The model under review builds one solid part; all positions refer to its coordinate system, in mm. A direction names the side the tool comes from. Coordinates: 2 decimals unless noted, no trailing zeros. Order: outer loops, then holes, each group sorted by start corner. A loop starts at its lowest first (then second) coordinate and runs counter-clockwise, first axis right, second up. Notation, with made-up numbers: M -12,-22.75 L 22,-22.75 A26 ccw 22,16.25 Z; hole C 69.25,74.5 d1. An arc over 180 degrees is marked long. Answer as CSV lines item,"result". Start each with the question number.
Q1. Consider section B-B on y = 7. Write out the cut boundary in (x, z), and give its area (3 significant figures).
Q2. The part is to be moulded in two halves that separate along Y. For faces 1 (the face through (23.846, 7.509, -29.58)), 2 (the face through (17, -2, -4)), 3 (the face through (0, 0, -100)), say which applies: +Y half, -Y half, draft (parallel to the pull), parting line (faces both ways), or undercut.
Q3. Consider section D-D on x = 0. Write out the cut boundary in (y, z).
Q4. Wall thickness on L1, parallel to Z at x = 23.5, y = 6.5; L2, parallel to X at y = -5.5, z = -8; L3, parallel to X at y = 15, z = -71: over which ranges is each line inside the solid? List them lowest first. Write a range as [from, to].
Q5. Consider section C-C on z = -31.5. Write out the cut boundary in (x, y), and give its area (3 significant figures).
Q6. For P1, Ø3, axis at y = -3, z = -1.5, coming from the +X side; P2, Ø2, axis at x = 20, z = -2, coming from the -Y side; P3, Ø1.2, axis at x = 17.5, y = -2.5, coming from the +Z side; P4, Ø1, axis at x = 7.5, y = 3, coming from the +Z side, all flat-tipped, find the tip position at first contact; note any pin that passes through.
Q7. Machinability: for faces 4 (the face through (11, -16, -60)), 5 (the face through (0, 0, 0)), 6 (the face through (17, 0, -2)), which of the approach directions +Z, -Z, +X, -X, +Y, -Y give a long, thin tool a straight path to every point of the face, cutting with its end or side? Answer none if there is none.
Q8. Consider section A-A on x = 13. Write out the cut boundary in (y, z).
from build123d import *

# Parameters (mm, degrees)
SKETCH_1_R          = 25
EXTRUDE_1_DEPTH     = 60
SKETCH_2_R          = 18
EXTRUDE_2_DEPTH     = 100
SKETCH_3_W          = 25
SKETCH_3_H          = 8
CUT_EXTRUDE_1_DEPTH = 4


with BuildPart() as part:
    # 草图1 → 凸台-拉伸1 (new body)
    with BuildSketch(Plane.XY):
        Circle(SKETCH_1_R)
    extrude(amount=-EXTRUDE_1_DEPTH)

    # 草图2 → 凸台-拉伸2 (add)
    with BuildSketch(Plane.XY):
        Circle(SKETCH_2_R)
    extrude(amount=-EXTRUDE_2_DEPTH)

    # 草图3 → 切除-拉伸1 (cut)
    with BuildSketch(Plane(origin=(0, 0, 0), x_dir=(1, 0, 0), z_dir=(0, 1, 0))):
        with Locations((22.5, 0)):
            Rectangle(SKETCH_3_W, SKETCH_3_H)
    extrude(amount=-CUT_EXTRUDE_1_DEPTH, mode=Mode.SUBTRACT)


solid = part.part
Evaluation:
1,outline,"M -24,-60 L -16.58,-60 L -16.58,-100 L 16.58,-100 L 16.58,-60 L 24,-60 L 24,0 L -24,0 Z"
1,area,"4,210 mm²"
2,face 1,"parting line"
2,face 2,"undercut"
2,face 3,"draft"
3,outline,"M -25,-60 L -18,-60 L -18,-100 L 18,-100 L 18,-60 L 25,-60 L 25,0 L -25,0 Z"
4,L1,"z = [-60, 0]"
4,L2,"x = [-24.39, 24.39]"
4,L3,"x = [-9.95, 9.95]"
5,outline,"C 0,0 d50"
5,area,"1,960 mm²"
6,P1,"stops at x = 24.68"
6,P2,"stops at y = -16.25"
6,P3,"stops at z = -4"
6,P4,"stops at z = 0"
7,face 4,"-Z"
7,face 5,"+Z, +X, -X, +Y, -Y"
7,face 6,"+Z, +X"
8,outline,"M -21.35,-60 L -12.45,-60 L -12.45,-100 L 12.45,-100 L 12.45,-60 L 21.35,-60 L 21.35,0 L 0,0 L 0,-4 L -4,-4 L -4,0 L -21.35,0 Z"
